from build123d import *

# Parameters (mm, degrees)
F1_DEPTH      = 38.1
F1_DEPTH_BACK = 38.1
F3_DEPTH      = 19.1664542539
F3_DEPTH_BACK = 14.5482714754
F4_R          = 16.5901380348
F5_DEPTH      = 38.1
F5_DEPTH_BACK = 38.1
F6_R          = 6.0434661234
F6_R_2        = 7.0228239136
F7_DEPTH      = 38.101
F7_DEPTH_BACK = 38.1


with BuildPart() as f1:
    # F0 (on Front) → F1 (new body, two sides)
    with BuildSketch(Plane.XZ) as f1_sk:
        with BuildLine():
            ThreePointArc((14.5467436103, 45.9329626612), (14.5471395086, 45.9996620138), (14.5472714754, 46.0663624108))
            ThreePointArc((14.5472714754, 46.0663624108), (-2.3090913892, 62.9227252754), (-19.1654542538, 46.0663624108))
            ThreePointArc((-19.1654542538, 46.0663624108), (-2.3757917862, 29.210131513), (14.5467436103, 45.9329626612))
        make_face()
        with BuildLine():
            ThreePointArc((14.5467436103, 45.9329626612), (-2.3757917862, 29.210131513), (-19.1654542538, 46.0663624108))
            Line((-19.1654542538, 46.0663624108), (-19.1654542538, -12.3536363244))
            Line((-19.1654542538, -12.3536363244), (14.0854548663, -12.3536363244))
            Line((14.0854548663, -12.3536363244), (14.5467436103, 45.9329626612))
        make_face()
    extrude(amount=F1_DEPTH)
    extrude(f1_sk.sketch, amount=-F1_DEPTH_BACK)

    # F2 (on Right) → F3 (cut, two sides)
    with BuildSketch(Plane.YZ) as f3_sk:
        Polygon((17.6418442279, 67.0483036786), (-23.7836372107, 66.8481811881), (-23.7836372107, -12.9865873605), (17.6418442279, -12.9865873605), align=None)
    extrude(amount=-F3_DEPTH, mode=Mode.SUBTRACT)
    extrude(f3_sk.sketch, amount=F3_DEPTH_BACK, mode=Mode.SUBTRACT)

    # F4 (on Front) → F5 (join, two sides)
    with BuildSketch(Plane.XZ) as f5_sk:
        with Locations((-2.3090913892, -12.3536363244)):
            Circle(F4_R)
    extrude(amount=F5_DEPTH)
    extrude(f5_sk.sketch, amount=-F5_DEPTH_BACK)

    # F6 (on Front) → F7 (cut, two sides)
    with BuildSketch(Plane.XZ) as f7_sk:
        with Locations((-2.3090913892, 46.0663624108)):
            Circle(F6_R)
        with Locations((-3.0018182006, -13.9700006694)):
            Circle(F6_R_2)
    extrude(amount=F7_DEPTH, mode=Mode.SUBTRACT)
    extrude(f7_sk.sketch, amount=-F7_DEPTH_BACK, mode=Mode.SUBTRACT)


solid = f1.part
CAD build for the part. Positions are in the model's coordinates, mm. Coordinates: 2 decimals unless noted, no trailing zeros. Write each loop counter-clockwise with the first axis right and the second up, starting at its lowest first coordinate (ties: lowest second). Pieces come first, ordered by that corner, then holes. Notation, with made-up numbers: (69.25, -13.5) - (74.25, -13.5) arc R9 cw to (74.25, 0.5) - close; hole circle Ø5 at (-26, 18.25). An arc over 180 degrees is marked (long way). Use a Markdown table: item, result. Add a question column.
Item 1: Mould opens along Y. For faces 1 (the face through (-3, 17.642, 33)), 2 (the face through (-3, -38.1, 18)), 3 (the face through (-19.165, 28, 17)), 4 (the face through (-3, -23.784, 26)) say: pulls with the +Y half, pulls with the -Y half, needs draft (parallel to the pull), parting line crosses it, or undercut.
Item 2: Band-saw the part on D-D, the plane y = -13. Give the cut face in (x, z), and give its area (3 significant figures).
Item 3: Band-saw the part on A-A, the plane y = -32.5. Give the cut face in (x, z).
Item 4: Band-saw the part on B-B, the plane x = -5. Give the cut face in (y, z).
Item 5: Band-saw the part on C-C, the plane z = -11. Give the cut face in (x, y).
Item 6: Drill centre lines: L1, parallel to Z at x = -2.5, y = -27.5; L2, parallel to Y at x = 4.5, z = 14.5; L3, parallel to Z at x = -0.5, y = 27. Where is each one in solid material? Low to high. Write a range as from..to.
Item 7: Flat gauge pins, fed straight in: pin 1 (2 mm diameter, centred on x = 5, y = 11, fed in from +Z); pin 2 (1.5 mm diameter, centred on x = -9, y = 9, fed in from +Z); pin 3 (1 mm diameter, centred on x = 9.5, y = -11, fed in from +Z). Where does each tip first touch, or does it go through?
Numbers:
| question | item | result |
|---|---|---|
| 1 | face 1 | undercut |
| 1 | face 2 | pulls with the -Y half |
| 1 | face 3 | needs draft |
| 1 | face 4 | undercut |
| 2 | outline | circle Ø33.18 at (-2.31, -12.35); hole circle Ø14.05 at (-3, -13.97) |
| 2 | area | 710 mm2 |
| 3 | outline | (-19.17, -12.35) - (-18.9, -12.35) arc R16.59 ccw (long way) to (14.1, -9.94) - (14.55, 45.93) arc R16.86 ccw to (14.55, 46.07) arc R16.86 ccw to (-19.17, 46.07) - close; hole circle Ø14.05 at (-3, -13.97); hole circle Ø12.09 at (-2.31, 46.07) |
| 4 | outline | (-38.1, -28.72) - (38.1, -28.72) - (38.1, -20.7) - (-38.1, -20.7) - close; (-38.1, -7.24) - (38.1, -7.24) - (38.1, 40.66) - (17.64, 40.66) - (17.64, 4.02) - (-23.78, 4.02) - (-23.78, 40.66) - (-38.1, 40.66) - close; (-38.1, 51.48) - (-23.78, 51.48) - (-23.78, 62.71) - (-38.1, 62.71) - close; (17.64, 51.48) - (38.1, 51.48) - (38.1, 62.71) - (17.64, 62.71) - close |
| 5 | outline | (-19.17, -38.1) - (-9.37, -38.1) - (-9.37, 38.1) - (-19.17, 38.1) - (-19.17, 17.64) - (-18.84, 17.64) - (-18.84, -23.78) - (-19.17, -23.78) - close; (3.36, -38.1) - (14.23, -38.1) - (14.23, 38.1) - (3.36, 38.1) - close |
| 6 | L1 | -28.94..-20.97, -6.97..40.03, 52.11..62.92 |
| 6 | L2 | -38.1..-23.78, 17.64..38.1 |
| 6 | L3 | -28.84..-20.53, -7.41..40.3, 51.83..62.83 |
| 7 | pin 1 | z = 2.99 |
| 7 | pin 2 | z = 3.14 |
| 7 | pin 3 | z = -0.22 |
